from build123d import *

# Parameters (mm, degrees)
SKETCH1_R               = 10
SKETCH1_R_2             = 5
BOSS_EXTRUDE2_DEPTH     = 2.5
CUT_EXTRUDE1_DEPTH      = 90.477650841
CUT_EXTRUDE1_DEPTH_BACK = 90.477650841
SKETCH3_R               = 4


with BuildPart() as part:
    # Sketch1 → Boss-Extrude2 (new, symmetric)
    with BuildSketch(Plane.XY):
        with BuildLine():
            Line((-39.119095531, -48.422064855), (-24.119095531, 6.577935145))
            ThreePointArc((-24.119095531, 6.577935145), (0, 25), (24.119095531, 6.577935145))
            Line((24.119095531, 6.577935145), (39.119095531, -48.422064855))
            ThreePointArc((39.119095531, -48.422064855), (34.867666932, -70.174841373), (15, -80))
            Line((15, -80), (-15, -80))
            ThreePointArc((-15, -80), (-34.867666932, -70.174841373), (-39.119095531, -48.422064855))
        make_face()
        Circle(SKETCH1_R, mode=Mode.SUBTRACT)
        with Locations((-15, -55)):
            Circle(SKETCH1_R_2, mode=Mode.SUBTRACT)
        with Locations((15, -55)):
            Circle(SKETCH1_R_2, mode=Mode.SUBTRACT)
    extrude(amount=BOSS_EXTRUDE2_DEPTH, both=True)

    # Sketch3 → Cut-Extrude1 (cut, two sides: drawn at the far end of the back side and taken through both)
    with BuildSketch(Plane.XY.offset(-CUT_EXTRUDE1_DEPTH_BACK)):
        with Locations((17.5, 0)):
            Circle(SKETCH3_R)
        with Locations((-17.5, 0)):
            Circle(SKETCH3_R)
    extrude(amount=CUT_EXTRUDE1_DEPTH + CUT_EXTRUDE1_DEPTH_BACK, mode=Mode.SUBTRACT)


solid = part.part
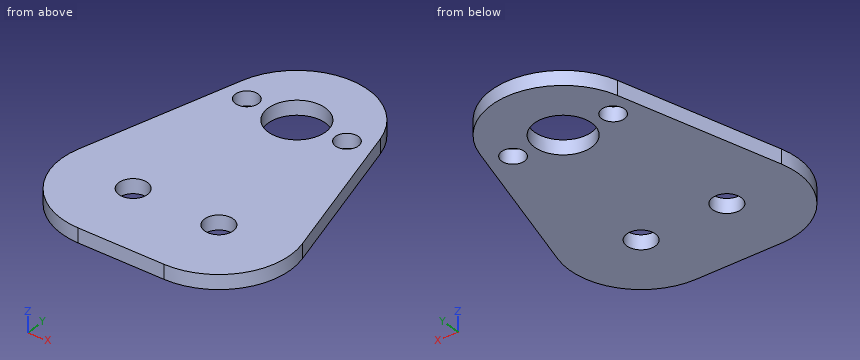
The listing builds one solid part. Answer for the finished solid, in the listing's coordinates (mm). Give positions to 0.01 mm unless a question says otherwise; leave off trailing zeros. Loops run counter-clockwise (first coordinate to the right, second up) from the corner with the lowest first, then second, coordinate; pieces in that order, holes last. Notation, with made-up numbers: (44, 44.5) - (82, 44.5) arc R9 ccw to (82, 54.5) - close; hole circle Ø9 at (-21, 2.25). An arc over 180 degrees is marked (long way). Answer as a JSON object with one key per item and string values.
1. Flat-ended cylindrical pins translate along their axes: pin 1 Ø1 at (x, z) = (18.5, 2) entering from +Y; pin 2 Ø5 at (x, y) = (-17.5, 0) entering from +Z. Find the tip coordinate at first contact, or state that the pin passes through.
Determined:
{"pin 1": "y = 17.35", "pin 2": "through"}
2. Find the intervals of material crossed by L1, parallel to Y at x = 0, z = -1.1; L2, parallel to Y at x = 15, z = -1.1; L3, parallel to Y at x = -17.5, z = 0.5, in increasing order. Write a range as [from, to].
Determined:
{"L1": "[-80, -10], [10, 25]", "L2": "[-80, -60], [-50, -3.12], [3.12, 20]", "L3": "[-79.87, -59.33], [-50.67, -4], [4, 17.85]"}
3. A cutting plane is placed at D-D (y = 0). Write down the section's boundary in (x, z).
Determined:
{"outline": "(-25.91, -2.5) - (-21.5, -2.5) - (-21.5, 2.5) - (-25.91, 2.5) - close; (-13.5, -2.5) - (-10, -2.5) - (-10, 2.5) - (-13.5, 2.5) - close; (10, -2.5) - (13.5, -2.5) - (13.5, 2.5) - (10, 2.5) - close; (21.5, -2.5) - (25.91, -2.5) - (25.91, 2.5) - (21.5, 2.5) - close"}
4. A cutting plane is placed at B-B (y = -55). Write down the section's boundary in (x, z), then the cut area to 3 significant figures.
Determined:
{"outline": "(-40, -2.5) - (-20, -2.5) - (-20, 2.5) - (-40, 2.5) - close; (-10, -2.5) - (10, -2.5) - (10, 2.5) - (-10, 2.5) - close; (20, -2.5) - (40, -2.5) - (40, 2.5) - (20, 2.5) - close", "area": "300 mm²"}
5. A cutting plane is placed at C-C (z = -1.4). Write down the section's boundary in (x, y).
Determined:
{"outline": "(-39.12, -48.42) arc R25 ccw to (-15, -80) - (15, -80) arc R25 ccw to (39.12, -48.42) - (24.12, 6.58) arc R25 ccw to (-24.12, 6.58) - close; hole circle Ø8 at (-17.5, 0); hole circle Ø10 at (-15, -55); hole circle Ø20 at (0, 0); hole circle Ø10 at (15, -55); hole circle Ø8 at (17.5, 0)"}
6. A cutting plane is placed at A-A (x = 0). Write down the section's boundary in (y, z), then the cut area to 3 significant figures.
Determined:
{"outline": "(-80, -2.5) - (-10, -2.5) - (-10, 2.5) - (-80, 2.5) - close; (10, -2.5) - (25, -2.5) - (25, 2.5) - (10, 2.5) - close", "area": "425 mm²"}
